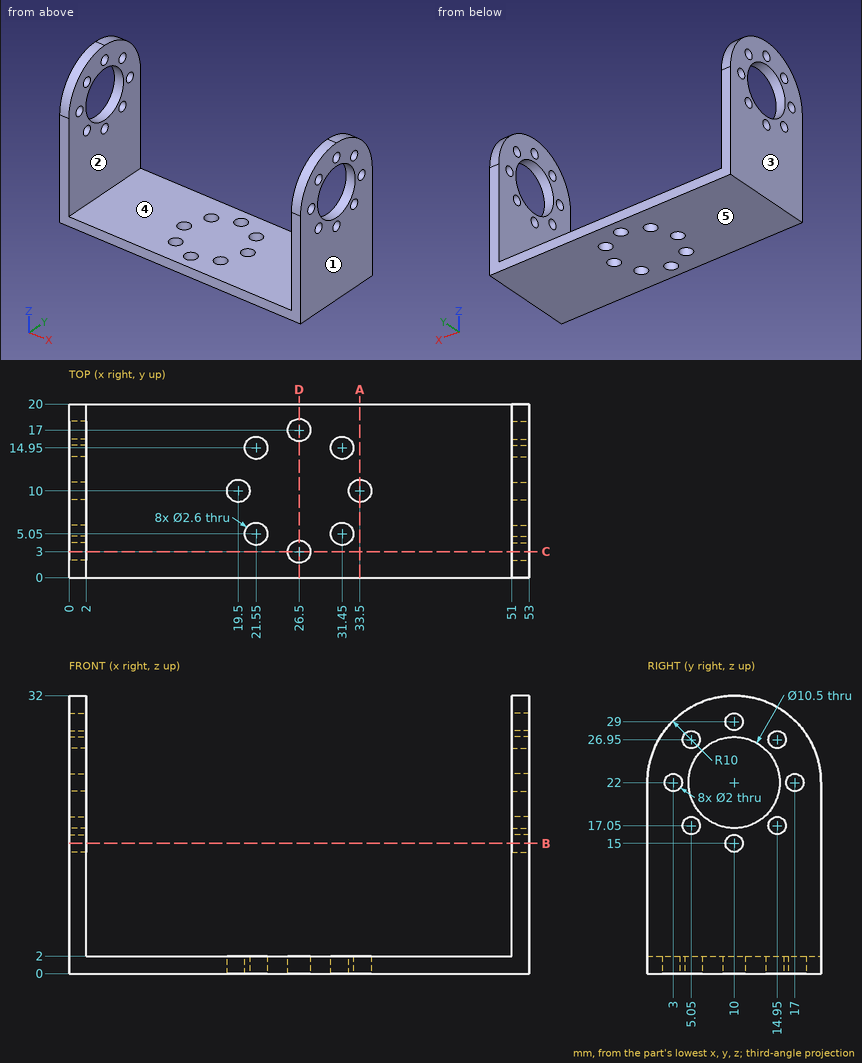
Check sheet for the drawn part. Datum: minimum x, y, z corner. Units: mm. A direction names the side the tool comes from. Coordinates: 2 decimals unless noted, no trailing zeros. Loops run counter-clockwise (first coordinate to the right, second up) from the corner with the lowest first, then second, coordinate; pieces in that order, holes last. Notation, with made-up numbers: (84, 88.25) -> (140, 88.25) arc R18 cw to (140, 111.25) -> close; hole circle Ø4 at (65.25, 84). An arc over 180 degrees is marked (long way). Answer as a JSON object with one key per item and string values. Group by question number.
Item 1: Scan lines: probe 1 along X at (y, z) = (8.25, 27); probe 2 along Z at (x, y) = (48, 17.75); probe 3 along Y at (x, z) = (52, 29). Record each from-to range of solid material in increasing order.
Item 2: Depth check by flat-ended pin: pin 1 (12 mm diameter, centred on y = 10, z = 22, fed in from +X); pin 2 (6 mm diameter, centred on y = 10.5, z = 21.5, fed in from +X); pin 3 (1.5 mm diameter, centred on x = 7.5, y = 12, fed in from +Z). Enter the tip coordinate at first touch or a pass-through.
Item 3: Mould release check, pull along X, two halves, no side actions. Record for the marked faces 1, 2 and 3: +X half, -X half, draft (parallel to the pull), parting line (faces both ways), or undercut.
Item 4: Sectioned sample at C-C on y = 3. Record the boundary of the cut face in (x, z).
Item 5: Sectioned sample at A-A on x = 33.5. Record the boundary of the cut face in (y, z).
Item 6: Tool access check on the marked faces 4 and 5. Record the directions out of +Z, -Z, +X, -X, +Y, -Y that give a thin tool (end or side, any length) a straight path to the whole face; none if there is none.
Item 7: Sectioned sample at B-B on z = 15. Record the boundary of the cut face in (x, y), plus the area to 3 significant figures.
Item 8: Sectioned sample at D-D on x = 26.5. Record the boundary of the cut face in (y, z), plus the area to 3 significant figures.
Evaluation:
{
 "1": {"probe 1": "x = 0 to 2, 51 to 53", "probe 2": "z = 0 to 2", "probe 3": "y = 2.86 to 9, 11 to 17.14"},
 "2": {"pin 1": "stops at x = 53", "pin 2": "passes through", "pin 3": "stops at z = 2"},
 "3": {"face 1": "+X half", "face 2": "undercut", "face 3": "-X half"},
 "4": {"outline": "(0, 0) -> (25.2, 0) -> (25.2, 2) -> (2, 2) -> (2, 21) -> (0, 21) -> close; (0, 23) -> (2, 23) -> (2, 29.14) -> (0, 29.14) -> close; (27.8, 0) -> (53, 0) -> (53, 21) -> (51, 21) -> (51, 2) -> (27.8, 2) -> close; (51, 23) -> (53, 23) -> (53, 29.14) -> (51, 29.14) -> close"},
 "5": {"outline": "(0, 0) -> (8.7, 0) -> (8.7, 2) -> (0, 2) -> close; (11.3, 0) -> (20, 0) -> (20, 2) -> (11.3, 2) -> close"},
 "6": {"face 4": "+Z, +Y, -Y", "face 5": "-Z, +X, -X, +Y, -Y"},
 "7": {"outline": "(0, 0) -> (2, 0) -> (2, 9) -> (0, 9) -> close; (0, 11) -> (2, 11) -> (2, 20) -> (0, 20) -> close; (51, 0) -> (53, 0) -> (53, 9) -> (51, 9) -> close; (51, 11) -> (53, 11) -> (53, 20) -> (51, 20) -> close", "area": "72.0 mm²"},
 "8": {"outline": "(0, 0) -> (1.7, 0) -> (1.7, 2) -> (0, 2) -> close; (4.3, 0) -> (15.7, 0) -> (15.7, 2) -> (4.3, 2) -> close; (18.3, 0) -> (20, 0) -> (20, 2) -> (18.3, 2) -> close", "area": "29.6 mm²"}
}
